Design review of the part built by this model. Coordinates are the model's own, in mm. A direction names the side the tool comes from. Coordinates: 2 decimals unless noted, no trailing zeros. Write each loop counter-clockwise with the first axis right and the second up, starting at its lowest first coordinate (ties: lowest second). Pieces come first, ordered by that corner, then holes.
Q1. Take a section at A-A (y = 11.5). Give the boundary of the cut face in (x, z), and give its area (3 significant figures).
Q2. Insertion check: pin 1 (3 mm diameter, centred on x = -10, z = 26, fed in from -Y); pin 2 (4 mm diameter, centred on x = -3, y = -3, fed in from +Z); pin 3 (3 mm diameter, centred on y = -3.5, z = 16.5, fed in from +X). Each pin has a flat end and moves straight along its axis. Give the tip position at first contact, or say it passes through.
Q3. Take a section at D-D (y = -0.5). Give the boundary of the cut face in (x, z), and give its area (3 significant figures).
Q4. Machinability: for faces 4 (the cylindrical face through (0.1, 3.7, -2.8)), 5 (the flat face through (-32, -5.9, 32)), 6 (the flat face through (-8, 1.6, 8)), which of the approach directions +Z, -Z, +X, -X, +Y, -Y give a long, thin tool a straight path to every point of the face, cutting with its end or side? Answer none if there is none.
Q5. Take a section at B-B (x = 0). State how many separate pieces and enclosed holes the cut face has, and give its area (3 significant figures).
Q6. Mouldability with a two-part tool opening along Z and no side actions: class faces 1 (the flat face through (-3, -6, 0)), 2 (the flat face through (-32, 5.9, 32)), 3 (the cylindrical face through (13.502, 6.245, 42.874)) as pulls with the +Z half, pulls with the -Z half, needs draft (parallel to the pull), parting line crosses it, or undercut.
Q7. For probe 1 along X at (y, z) = (6.5, 0) (3 decimals); probe 2 along X at (y, z) = (-3, 0.5) (3 decimals); probe 3 along Z at (x, y) = (6.5, -0.5), list the stretches that pass through material, from the lowest coordinate up.
```python
from build123d import *

# Parameters (mm, degrees)
SKETCH1_R           = 48.1
BOSS_EXTRUDE2_DEPTH = 5.9
SKETCH2_R           = 44.95
BOSS_EXTRUDE3_DEPTH = 0.7
SKETCH5_R           = 40.15
CUT_EXTRUDE1_DEPTH  = 5
SKETCH8_R           = 9.95
CUT_EXTRUDE2_DEPTH  = 69.516129488
SKETCH8_4_R         = 9.5
BOSS_EXTRUDE4_DEPTH = 11.6
SKETCH9_R           = 8.5
SKETCH10_R          = 7.95
CUT_EXTRUDE3_REACH  = 72.847
SKETCH11_R          = 2.8


# Read off the part's stored shape, not the designer's step: Loft2, Loft3
with BuildPart() as part:
    # Sketch1 → Boss-Extrude2 (new body)
    with BuildSketch(Plane(origin=(0, 0, 0), x_dir=(1, 0, 0), z_dir=(0, 1, 0))):
        with Locations(Location((0, 0, 0), (0, 0, 270))):
            Circle(SKETCH1_R)
    boss_extrude2 = extrude(amount=BOSS_EXTRUDE2_DEPTH)

    # Sketch2 → Boss-Extrude3 (add)
    with BuildSketch(Plane(origin=(0, 5.9, 0), x_dir=(1, 0, 0), z_dir=(0, 1, 0))):
        with Locations(Location((0, 0, 0), (0, 0, 270))):
            Circle(SKETCH2_R)
    boss_extrude3 = extrude(amount=BOSS_EXTRUDE3_DEPTH)

    # Sketch5 → Cut-Extrude1 (cut)
    with BuildSketch(Plane(origin=(0, 6.6, 0), x_dir=(1, 0, 0), z_dir=(0, 1, 0))):
        with Locations(Location((0, 0, 0), (0, 0, 270))):
            Circle(SKETCH5_R)
    cut_extrude1 = extrude(amount=-CUT_EXTRUDE1_DEPTH, mode=Mode.SUBTRACT)

    # Loft2 outline → Loft2 (revolve)
    with BuildSketch(Plane.XY):
        Polygon((40.15, 6.6), (39.4, 1.6), (40.15, 1.6), align=None)
    revolve(axis=Axis((0, 0, 0), (0, 1, 0)))

    # Mirror2: Boss-Extrude2, Boss-Extrude3, Cut-Extrude1 across Top Plane
    add(boss_extrude2.mirror(Plane(origin=(0, 0, 0), x_dir=(1, 0, 0), z_dir=(0, 1, 0))))
    add(boss_extrude3.mirror(Plane(origin=(0, 0, 0), x_dir=(1, 0, 0), z_dir=(0, 1, 0))))
    add(cut_extrude1.mirror(Plane(origin=(0, 0, 0), x_dir=(1, 0, 0), z_dir=(0, 1, 0))), mode=Mode.SUBTRACT)

    # Loft3 outline → Loft3 (revolve)
    with BuildSketch(Plane.XY):
        Polygon((40.15, -1.6), (39.4, -1.6), (40.15, -6.6), align=None)
    revolve(axis=Axis((0, 0, 0), (0, 1, 0)))

    # Sketch8 → Cut-Extrude2 (cut, through all)
    with BuildSketch(Plane(origin=(0, 1.6, 0), x_dir=(1, 0, 0), z_dir=(0, 1, 0))):
        with Locations(Location((0, -25, 0), (0, 0, 270))):
            Circle(SKETCH8_R)
        with Locations(Location((-23.776412907, -7.725424859, 0), (0, 0, 270))):
            Circle(SKETCH8_R)
        with Locations(Location((-14.694631307, 20.225424859, 0), (0, 0, 270))):
            Circle(SKETCH8_R)
        with Locations(Location((14.694631307, 20.225424859, 0), (0, 0, 270))):
            Circle(SKETCH8_R)
        with Locations(Location((23.776412907, -7.725424859, 0), (0, 0, 270))):
            Circle(SKETCH8_R)
    extrude(amount=-CUT_EXTRUDE2_DEPTH, mode=Mode.SUBTRACT)

    # Sketch8<4> → Boss-Extrude4 (add)
    with BuildSketch(Plane(origin=(0, 1.6, 0), x_dir=(1, 0, 0), z_dir=(0, 1, 0))):
        with Locations(Location((0, 0, 0), (0, 0, 270))):
            Circle(SKETCH8_4_R)
    extrude(amount=BOSS_EXTRUDE4_DEPTH)

    # Sketch9 → Loft4 section 0
    with BuildSketch(Plane.XZ.offset(1.6)):
        Circle(SKETCH9_R)
    # Sketch10 → Loft4 section 1
    with BuildSketch(Plane(origin=(0, -6, 0), x_dir=(-1, 0, 0), z_dir=(0, -1, 0))):
        Circle(SKETCH10_R)
    loft()

    # Sketch11 → Cut-Extrude3 (cut, up to next)
    with BuildSketch(Plane(origin=(0, 13.2, 0), x_dir=(1, 0, 0), z_dir=(0, 1, 0)), mode=Mode.PRIVATE) as cut_extrude3_sk1:
        with Locations(Location((0, 0, 0), (0, 0, 270))):
            Circle(SKETCH11_R)
    cut_extrude3_tool1 = extrude(cut_extrude3_sk1.sketch, amount=-CUT_EXTRUDE3_REACH, mode=Mode.PRIVATE) & part.part
    add(cut_extrude3_tool1.solids().sort_by_distance((0, 13.2, 0))[0], mode=Mode.SUBTRACT)


solid = part.part
```
Response:
1. outline: circle Ø19 at (0, 0); hole circle Ø5.6 at (0, 0)
1. area: 259 mm2
2. pin 1: stops at y = -1.6
2. pin 2: stops at z = 48.09
2. pin 3: stops at x = 45.7
3. outline: circle Ø96.2 at (0, 0); hole circle Ø19.9 at (-23.78, 7.73); hole circle Ø19.9 at (-14.69, -20.23); hole circle Ø19.9 at (0, 25); hole circle Ø5.6 at (0, 0); hole circle Ø19.9 at (14.69, -20.23); hole circle Ø19.9 at (23.78, 7.73)
3. area: 5,690 mm2
4. face 4: +Y, -Y
4. face 5: -Y
4. face 6: +Y
5. separate pieces: 3
5. enclosed holes: 0
5. area: 587 mm2
6. face 1: undercut
6. face 2: needs draft
6. face 3: parting line crosses it
7. probe 1: x = -44.95 to -40.135, -9.5 to -2.8, 2.8 to 9.5, 40.135 to 44.95
7. probe 2: x = -48.097 to -39.607, -8.31 to -2.755, 2.755 to 8.31, 39.607 to 48.097
7. probe 3: z = -47.66 to -25.87, -14.58 to 17.47, 32.53 to 47.66
